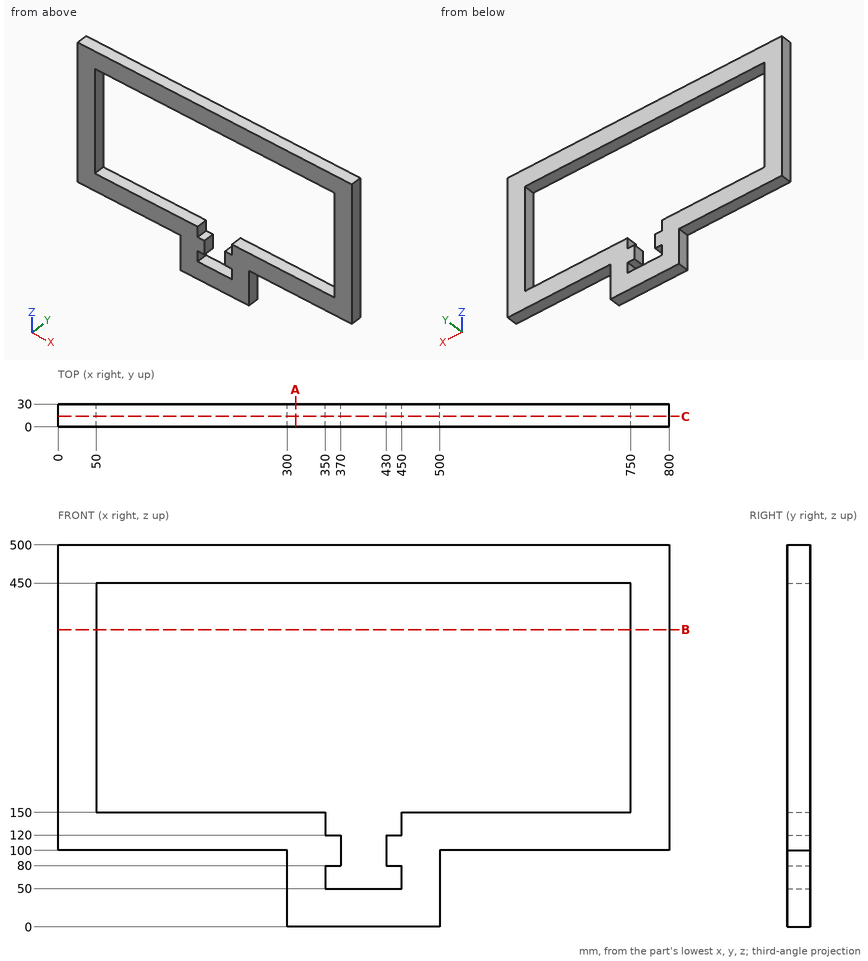
The drawing under review shows one solid part. Ordinate dimensions are in mm from its lowest x, y, z. Round coordinates to 2 decimals unless told otherwise and drop trailing zeros. Order: outer loops, then holes, each group sorted by start corner. A loop starts at its lowest first (then second) coordinate and runs counter-clockwise, first axis right, second up. Notation, with made-up numbers: (34, 63) -> (59, 63) arc R12 cw to (59, 82) -> close; hole circle Ø5 at (-37, 29.5). An arc over 180 degrees is marked (long way). Return JSON: item names as keys, results as strings.
1. Take a section at A-A (x = 311). Write out the cut boundary in (y, z).
Answer block:
{"outline": "(0, 0) -> (30, 0) -> (30, 150) -> (0, 150) -> close; (0, 450) -> (30, 450) -> (30, 500) -> (0, 500) -> close"}
2. Insertion check: P1, Ø12, axis at y = 10, z = 86, coming from the +X side; P2, Ø15, axis at y = 12.5, z = 328.5, coming from the -X side; P3, Ø9, axis at y = 7.5, z = 65.5, coming from the -X side; P4, Ø1, axis at x = 657, y = 13.5, coming from the -Z side. Each pin has a flat end and moves straight along its axis. Give the tip position at first contact, or say it passes through.
Answer block:
{"P1": "stops at x = 500", "P2": "stops at x = 0", "P3": "stops at x = 300", "P4": "stops at z = 100"}
3. Take a section at B-B (z = 389). Write out the cut boundary in (x, y), then the cut area to 3 significant figures.
Answer block:
{"outline": "(0, 0) -> (50, 0) -> (50, 30) -> (0, 30) -> close; (750, 0) -> (800, 0) -> (800, 30) -> (750, 30) -> close", "area": "3,000 mm²"}
4. For L1, parallel to Z at x = 360, y = 2.75; L2, parallel to X at y = 28.5, z = 367; L3, parallel to Z at x = 214, y = 15.75, list the stretches that pass through material, from the lowest coordinate up. Write a range as [from, to].
Answer block:
{"L1": "z = [0, 50], [80, 120], [450, 500]", "L2": "x = [0, 50], [750, 800]", "L3": "z = [100, 150], [450, 500]"}
5. Take a section at C-C (y = 13.75). Write out the cut boundary in (x, z), then the cut area to 3 significant figures.
Answer block:
{"outline": "(0, 100) -> (300, 100) -> (300, 0) -> (500, 0) -> (500, 100) -> (800, 100) -> (800, 500) -> (0, 500) -> close; hole (50, 150) -> (350, 150) -> (350, 120) -> (370, 120) -> (370, 80) -> (350, 80) -> (350, 50) -> (450, 50) -> (450, 80) -> (430, 80) -> (430, 120) -> (450, 120) -> (450, 150) -> (750, 150) -> (750, 450) -> (50, 450) -> close", "area": "122,000 mm²"}
